Drawing for the job (mm, zero at the part's lowest x, y, z). Round coordinates to 2 decimals unless told otherwise and drop trailing zeros. Loops run counter-clockwise (first coordinate to the right, second up) from the corner with the lowest first, then second, coordinate; pieces in that order, holes last.
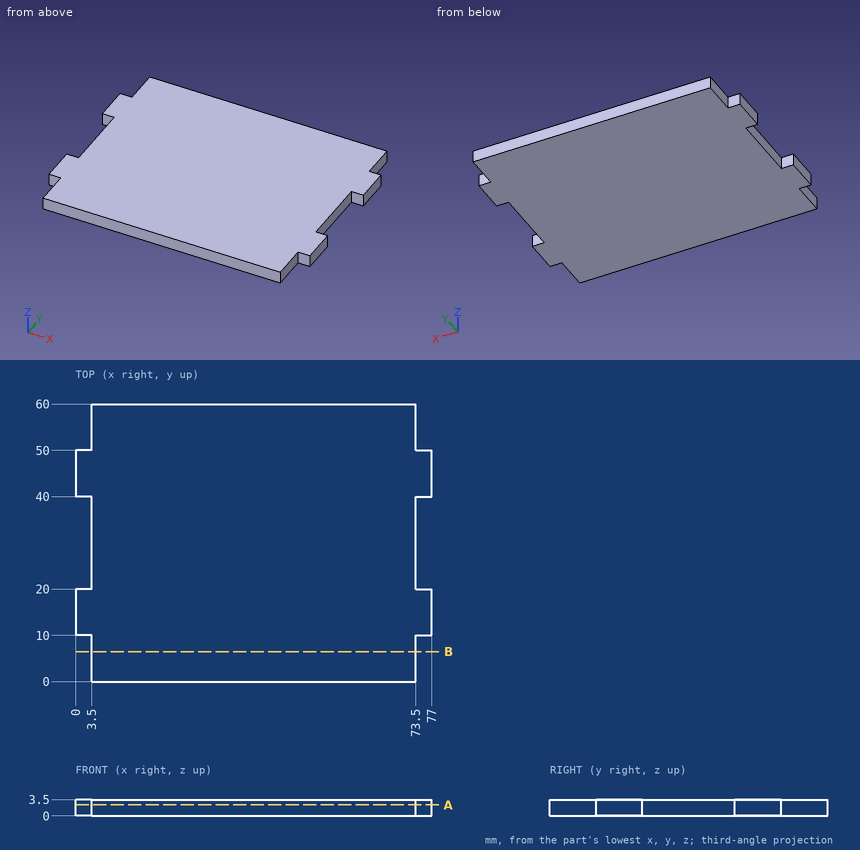
Q1. Probe line 1 (X direction, y = 21.5, z = 0.5). List the from-to ranges inside material, lowest first.
Q2. Slice it at B-B on y = 6.5. Give the cut face in (x, z).
Q3. Slice it at A-A on z = 2.35. Give the cut face in (x, y), plus the area to 3 significant figures.
Q4. Flat gauge pins, fed straight in: P1, Ø1.8, axis at y = 52.5, z = 2.5, coming from the +X side; P2, Ø1.8, axis at x = 74.5, z = 2.5, coming from the +Y side; P3, Ø1.8, axis at y = 2.5, z = 1.5, coming from the -X side. Where does each tip first touch, or does it go through?
Reply:
1. line 1: x = 3.5 to 73.5
2. outline: (3.5, 0) - (73.5, 0) - (73.5, 3.5) - (3.5, 3.5) - close
3. outline: (0, 10) - (3.5, 10) - (3.5, 0) - (73.5, 0) - (73.5, 10) - (77, 10) - (77, 20) - (73.5, 20) - (73.5, 40) - (77, 40) - (77, 50) - (73.5, 50) - (73.5, 60) - (3.5, 60) - (3.5, 50) - (0, 50) - (0, 40) - (3.5, 40) - (3.5, 20) - (0, 20) - close
3. area: 4,340 mm2
4. P1: stops at x = 73.5
4. P2: stops at y = 50
4. P3: stops at x = 3.5
